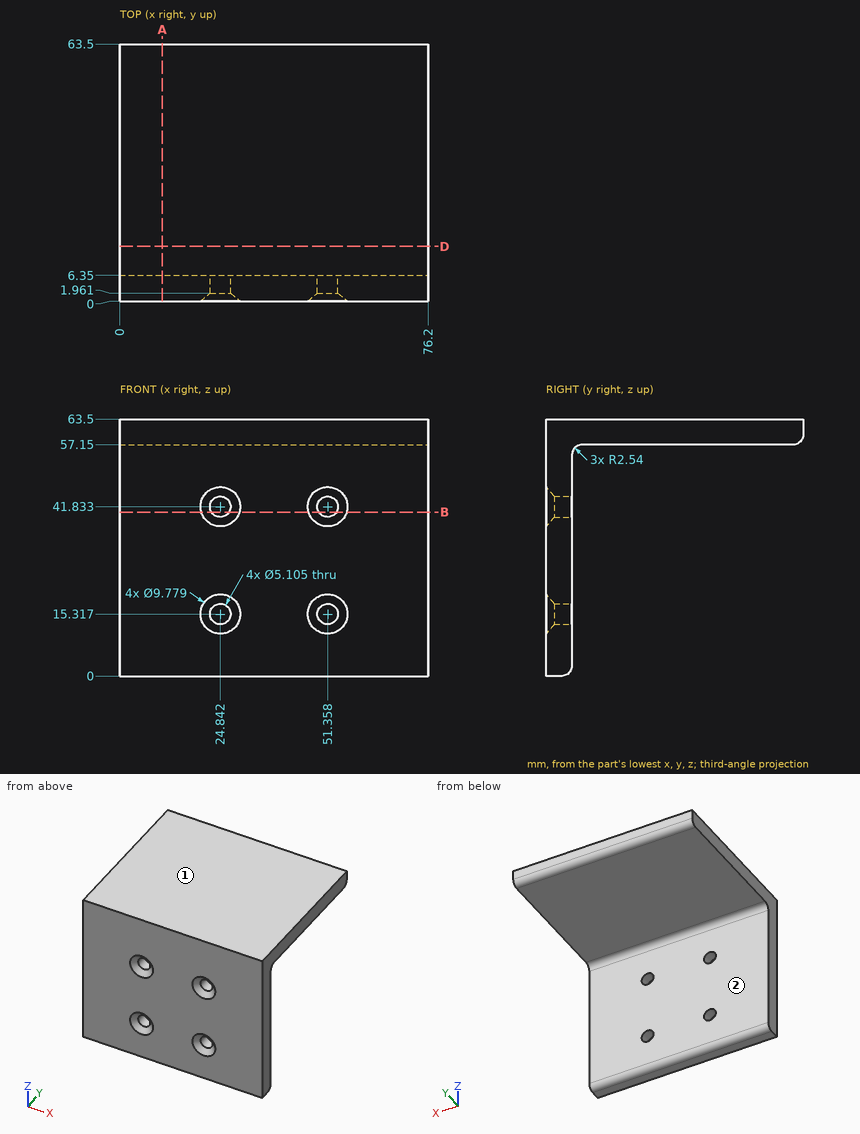
Answer from the drawing. Dimensions are ordinates in mm from the lowest x, y and z of the part. A direction names the side the tool comes from. Give positions to 0.01 mm unless a question says otherwise; leave off trailing zeros. Order: outer loops, then holes, each group sorted by start corner. A loop starts at its lowest first (then second) coordinate and runs counter-clockwise, first axis right, second up. Notation, with made-up numbers: (68, 0) - (105, 0) arc R12 cw to (105, 19) - close; hole circle Ø2 at (-34, 52.25). An arc over 180 degrees is marked (long way). One line per item, written item: value. Start each with the question number.
1) Find the intervals of material crossed by L1, parallel to Z at x = 27, y = 4.5 (1 decimal); L2, parallel to Z at x = 47, y = 17.5; L3, parallel to Y at x = 41, z = 35.5, in increasing order.
2) A cutting plane is placed at A-A on x = 10.5. Give the vertices of the cut face in (y, z), then the cut area to 3 significant figures.
3) A cutting plane is placed at D-D on y = 13.5. Give the vertices of the cut face in (x, z), then the cut area to 3 significant figures.
4) Given pin 1 Ø6.5 at (x, z) = (24.84, 41.83) entering from +Y; pin 2 Ø10 at (y, z) = (16, 22) entering from -X; pin 3 Ø8 at (x, z) = (24.84, 15.32) entering from -Y; pin 4 Ø5 at (x, y) = (45, 39) entering from -Z, each flat-ended and moving along its own axis, determine where each tip first touches the part or whether it passes through.
5) A tool of negligible diameter and unlimited length cuts with its end or side. For the marked faces 1 and 2, from which of +Z, -Z, +X, -X, +Y, -Y can it reach the whole face along a straight path? Write none if from no direction.
6) A cutting plane is placed at B-B on z = 40.5. State how many separate pieces and enclosed holes the cut face has.
Answer sheet:
1. L1: z = 0.1 to 14, 16.7 to 40.5, 43.2 to 63.5
1. L2: z = 57.15 to 63.5
1. L3: y = 0 to 6.35
2. outline: (0, 0) - (3.81, 0) arc R2.54 ccw to (6.35, 2.54) - (6.35, 54.61) arc R2.54 cw to (8.89, 57.15) - (60.96, 57.15) arc R2.54 ccw to (63.5, 59.69) - (63.5, 63.5) - (0, 63.5) - close
2. area: 765 mm2
3. outline: (0, 57.15) - (76.2, 57.15) - (76.2, 63.5) - (0, 63.5) - close
3. area: 484 mm2
4. pin 1: stops at y = 6.35
4. pin 2: passes through
4. pin 3: stops at y = 0.74
4. pin 4: stops at z = 57.15
5. face 1: +Z, +X, -X, +Y, -Y
5. face 2: -Z, +X, -X, +Y
6. separate pieces: 3
6. enclosed holes: 0
